from build123d import *

# Parameters (mm, degrees)
SKETCH_W        = 29.95
SKETCH_H        = 21.5
PAD_DEPTH       = 15
POCKET_DEPTH    = 21.501
SKETCH002_R     = 5
POCKET001_DEPTH = 30.001
POCKET002_DEPTH = 7
POCKET003_DEPTH = 7
PAD001_DEPTH    = 5
CHAMFER_SIZE    = 9.049
POCKET004_DEPTH = 18.8
SKETCH007_R     = 2.2
POCKET005_DEPTH = 2.701
SKETCH008_R     = 1.65
POCKET006_DEPTH = 10
POCKET007_DEPTH = 3
FILLET_R        = 2.2
FILLET001_R     = 3
CHAMFER001_SIZE = 0.75
CHAMFER002_SIZE = 0.5
CHAMFER003_SIZE = 0.5


with BuildPart() as part:
    # Sketch → Pad (new body, symmetric)
    with BuildSketch(Plane.XY):
        with Locations((0, -1.25)):
            Rectangle(SKETCH_W, SKETCH_H)
    extrude(amount=PAD_DEPTH, both=True)

    # Sketch001 (on Face1 of Pad) → Pocket (cut, through all)
    with BuildSketch(Plane(origin=(0, 9.5, 0), x_dir=(-1, 0, 0), z_dir=(0, 1, 0))):
        with BuildLine():
            Line((14.975, 1.5), (14.975, 5))
            Line((14.975, 5), (-8.224983, 5))
            ThreePointArc((-8.224983, 5), (-9.975, 3.25), (-8.224983, 1.5))
            Line((14.975, 1.5), (-8.224983, 1.5))
        make_face()
    extrude(amount=-POCKET_DEPTH, mode=Mode.SUBTRACT)

    # Sketch002 (on Face4 of Pocket) → Pocket001 (cut, through all)
    with BuildSketch(Plane.XY.offset(15)):
        Circle(SKETCH002_R)
    extrude(amount=-POCKET001_DEPTH, mode=Mode.SUBTRACT)

    # Sketch003 (on Face4 of Pocket001) → Pocket002 (cut)
    with BuildSketch(Plane.XY.offset(15)):
        Polygon((7.534421, 0), (3.767211, 6.525), (-3.767211, 6.525), (-7.534421, 0), (-3.767211, -6.525), (3.767211, -6.525), align=None)
    extrude(amount=-POCKET002_DEPTH, mode=Mode.SUBTRACT)

    # Sketch004 (on Face2 of Pocket002) → Pocket003 (cut)
    with BuildSketch(Plane(origin=(0, 0, -15), x_dir=(1, 0, 0), z_dir=(0, 0, -1))):
        Polygon((7.534421, 0), (3.767211, 6.525), (-3.767211, 6.525), (-7.534421, 0), (-3.767211, -6.525), (3.767211, -6.525), align=None)
    extrude(amount=-POCKET003_DEPTH, mode=Mode.SUBTRACT)

    # Sketch005 (on Face10 of Pocket003) → Pad001 (new body)
    with BuildSketch(Plane.XZ.offset(12)):
        Polygon((-14.975, 1.4), (-19.459732, 1.4), (-24.025, -1.235759), (-24.025, -9.92488), (-19.459732, -12.560639), (-14.975, -12.560639), align=None)
        Polygon((14.975, 1.4), (14.975, -12.560639), (19.459732, -12.560639), (24.025, -9.92488), (24.025, -1.235759), (19.459732, 1.4), align=None)
    extrude(amount=-PAD001_DEPTH)

    # Chamfer
    chamfer_edges = [part.edges().sort_by_distance(p)[0] for p in [
        (-14.975, -7, -5.580319),
        (14.975, -7, -5.580319),
    ]]
    chamfer(chamfer_edges, length=CHAMFER_SIZE)

    # Sketch006 (on Face7 of Chamfer) → Pocket004 (cut)
    with BuildSketch(Plane(origin=(0, 9.5, 0), x_dir=(-1, 0, 0), z_dir=(0, 1, 0))):
        Polygon((22.025, -7.61548), (22.025, -3.54516), (18.5, -1.510001), (14.975, -3.54516), (14.975, -7.61548), (18.5, -9.650639), align=None)
        Polygon((-18.5, -9.650639), (-14.975, -7.61548), (-14.975, -3.54516), (-18.5, -1.510001), (-22.025, -3.54516), (-22.025, -7.61548), align=None)
    extrude(amount=-POCKET004_DEPTH, mode=Mode.SUBTRACT)

    # Sketch007 (on Face36 of Pocket004) → Pocket005 (cut, through all)
    with BuildSketch(Plane(origin=(0, -9.3, 0), x_dir=(-1, 0, 0), z_dir=(0, 1, 0))):
        with Locations((-18.5, -5.58032)):
            Circle(SKETCH007_R)
        with Locations((18.5, -5.58032)):
            Circle(SKETCH007_R)
    extrude(amount=-POCKET005_DEPTH, mode=Mode.SUBTRACT)

    # Sketch008 (on Face23 of Pocket005) → Pocket006 (cut)
    with BuildSketch(Plane.XY.offset(15)):
        with Locations((-11.254711, 0)):
            Circle(SKETCH008_R)
    extrude(amount=-POCKET006_DEPTH, mode=Mode.SUBTRACT)

    # Sketch009 (on Face26 of Pocket006) → Pocket007 (cut)
    with BuildSketch(Plane(origin=(0, 0, 5), x_dir=(1, 0, 0), z_dir=(0, 0, -1))):
        Polygon((-9.652564, -2.775), (-8.050417, 0), (-9.652564, 2.775), (-12.856858, 2.775), (-14.459005, 0), (-12.856858, -2.775), align=None)
    extrude(amount=-POCKET007_DEPTH, mode=Mode.SUBTRACT)

    # Fillet
    fillet_edges = [part.edges().sort_by_distance(p)[0] for p in [
        (-14.975, -1.25, -15),
        (14.975, -1.25, -15),
        (-14.975, -1.25, 15),
        (14.975, -1.25, 15),
    ]]
    fillet(fillet_edges, radius=FILLET_R)

    # Fillet001
    fillet001_edges = [part.edges().sort_by_distance(p)[0] for p in [
        (24.025, -9.5, -9.92488),
        (19.459732, -7.217866, -12.560639),
        (24.025, -9.5, -1.235759),
        (-19.459732, -7.217866, -12.560639),
        (-24.025, -9.5, -9.92488),
        (-24.025, -9.5, -1.235759),
        (-19.459732, -7.217866, 1.4),
        (19.459732, -7.217866, 1.4),
    ]]
    fillet(fillet001_edges, radius=FILLET001_R)

    # Chamfer001
    chamfer001_edges = [part.edges().sort_by_distance(p)[0] for p in [
        (-5.650816, -3.2625, -15),
        (0, -6.525, -15),
        (5.650816, -3.2625, -15),
        (5.650816, 3.2625, -15),
        (0, 6.525, -15),
        (-5.650816, 3.2625, -15),
        (-5.650816, 3.2625, 15),
        (0, 6.525, 15),
        (5.650816, 3.2625, 15),
        (5.650816, -3.2625, 15),
        (0, -6.525, 15),
        (-5.650816, -3.2625, 15),
    ]]
    chamfer(chamfer001_edges, length=CHAMFER001_SIZE)

    # Chamfer002
    chamfer002_edges = [part.edges().sort_by_distance(p)[0] for p in [
        (-16.7375, 0.2865, -8.63306),
        (-16.7375, 0.2865, -2.52758),
        (-20.2625, -3.2385, -2.52758),
        (-20.2625, -3.2385, -8.63306),
        (-22.025, -5.001, -5.58032),
        (16.7375, 0.2865, -2.52758),
        (16.7375, 0.2865, -8.63306),
        (20.2625, -3.2385, -8.63306),
        (22.025, -5.001, -5.58032),
        (20.2625, -3.2385, -2.52758),
    ]]
    chamfer(chamfer002_edges, length=CHAMFER002_SIZE)

    # Chamfer003
    chamfer003_edges = [part.edges().sort_by_distance(p)[0] for p in [
        (-16.3, -12, -5.58032),
        (20.7, -12, -5.58032),
    ]]
    chamfer(chamfer003_edges, length=CHAMFER003_SIZE)


solid = part.part
The listing builds one solid part. Answer for the finished solid, in the listing's coordinates (mm). A direction names the side the tool comes from. Give positions to 0.01 mm unless a question says otherwise; leave off trailing zeros. Write each loop counter-clockwise with the first axis right and the second up, starting at its lowest first coordinate (ties: lowest second). Pieces come first, ordered by that corner, then holes. Notation, with made-up numbers: (-29, 0) - (-5, 0) arc R16 cw to (-5, 21) - close; hole circle Ø7 at (-1.75, 81). An arc over 180 degrees is marked (long way). One line per question, with ' | ' between items. Start each with the question number.
1. Section C-C, the plane x = -10.5 is taken. Determine the outline of the cut face in (y, z) (3 decimals).
2. Section A-A, the plane x = 0 is taken. Determine the outline of the cut face in (y, z) (3 decimals).
3. Section D-D, the plane y = -10 is taken. Count the separate pieces of the cut face and the enclosed holes in it, then the cut area to 3 significant figures.
4. Straight lines are drawn through the part: line 1 (Z direction, x = -8, y = 4.25); line 2 (Z direction, x = 18.5, y = -10.1); line 3 (Y direction, x = -3.5, z = -12.5) (3 decimals). For each, find the intervals that lie inside material, in ascending order.
5. Section B-B, the plane z = 9.5 is taken. Determine the outline of the cut face in (x, y) (3 decimals), then the cut area to 3 significant figures.
6. Given P1, Ø2, axis at x = -18.5, z = -6, coming from the +Y side; P2, Ø3, axis at x = 15.5, y = 5.5, coming from the -Z side; P3, Ø2.5, axis at y = -1.5, z = 7.5, coming from the -X side (3 decimals); P4, Ø5, axis at y = -7.5, z = -12, coming from the +X side, each flat-ended and moving along its own axis, determine where each tip first touches the part or whether it passes through.
7. Determine the mould class of faces 1 (the face through (14.348, -1.099, 14.338)), 2 (the face through (-6, 3.4, -14.62)), 3 (the face through (0, 9.5, 0)) for opening direction X: +X half, -X half, draft (parallel to the pull), parting line (faces both ways), or undercut.
8. For faces 4 (the face through (-5.624, -3.308, -11.169)), 5 (the face through (16.76, -0.07, -2.25)), 6 (the face through (-11, -2.775, 6)), 7 (the face through (-21.574, -4.55, -8.78)), 8 (the face through (-14.975, 3, -6)), determine the directions among +Z, -Z, +X, -X, +Y, -Y from which every point of the face is accessible in a straight line to the end or side of a thin tool.
Result:
1) outline: (-12, -15) - (9.5, -15) - (9.5, 1.5) - (-12, 1.5) - close; (-12, 5) - (-2.775, 5) - (-2.775, 8) - (-1.467, 8) - (-1.467, 15) - (-12, 15) - close; (1.467, 8) - (2.775, 8) - (2.775, 5) - (9.5, 5) - (9.5, 15) - (1.467, 15) - close
2) outline: (-12, -15) - (-7.275, -15) - (-6.525, -14.25) - (-6.525, -8) - (-5, -8) - (-5, 1.5) - (-12, 1.5) - close; (-12, 5) - (-5, 5) - (-5, 8) - (-6.525, 8) - (-6.525, 14.25) - (-7.275, 15) - (-12, 15) - close; (5, -8) - (6.525, -8) - (6.525, -14.25) - (7.275, -15) - (9.5, -15) - (9.5, 1.5) - (5, 1.5) - close; (5, 5) - (9.5, 5) - (9.5, 15) - (7.275, 15) - (6.525, 14.25) - (6.525, 8) - (5, 8) - close
3) separate pieces: 1 | enclosed holes: 2 | area: 1,000 mm2
4) line 1: z = -15 to 1.5, 5 to 15 | line 2: z = -12.56 to -7.78, -3.38 to 1.4 | line 3: y = -12 to -6.525, 6.525 to 9.5
5) outline: (-14.975, -12) - (14.975, -12) - (14.975, 9.5) - (-14.975, 9.5) - close; hole circle Ø3.3 at (-11.255, 0); hole (-7.534, 0) - (-3.767, -6.525) - (3.767, -6.525) - (7.534, 0) - (3.767, 6.525) - (-3.767, 6.525) - close | area: 488 mm2
6) P1: passes through | P2: stops at z = -14.63 | P3: stops at x = -14.975 | P4: stops at x = 23.73
7) face 1: +X half | face 2: undercut | face 3: draft
8) face 4: -Z | face 5: +X, +Y | face 6: none | face 7: +Z, -Z, -X, +Y | face 8: +Y
